```python
from build123d import *

# Parameters (mm, degrees)
SCHIZZO2_R                   = 55.0225
SCHIZZO2_R_2                 = 40.0225
ESTRUSIONE_ESTRUSIONE1_DEPTH = 10
SCHIZZO2_3_R                 = 40.0225
SCHIZZO2_3_R_2               = 25.0225
ESTRUSIONE_ESTRUSIONE2_DEPTH = 15
SCHIZZO2_4_R                 = 25.0225
SCHIZZO2_4_R_2               = 5
ESTRUSIONE_ESTRUSIONE3_DEPTH = 20


with BuildPart() as part:
    # Schizzo2 → Estrusione-Estrusione1 (new body)
    with BuildSketch(Plane(origin=(0, 0, 0), x_dir=(1, 0, 0), z_dir=(0, 1, 0))):
        with Locations(Location((0, 0, 0), (0, 0, 270))):
            Circle(SCHIZZO2_R)
        with Locations(Location((0, 0, 0), (0, 0, 270))):
            Circle(SCHIZZO2_R_2, mode=Mode.SUBTRACT)
    extrude(amount=ESTRUSIONE_ESTRUSIONE1_DEPTH)

    # Schizzo2_3 → Estrusione-Estrusione2 (add)
    with BuildSketch(Plane(origin=(0, 0, 0), x_dir=(1, 0, 0), z_dir=(0, 1, 0))):
        with Locations(Location((0, 0, 0), (0, 0, 270))):
            Circle(SCHIZZO2_3_R)
        with Locations(Location((0, 0, 0), (0, 0, 270))):
            Circle(SCHIZZO2_3_R_2, mode=Mode.SUBTRACT)
    extrude(amount=ESTRUSIONE_ESTRUSIONE2_DEPTH)

    # Schizzo2_4 → Estrusione-Estrusione3 (add)
    with BuildSketch(Plane(origin=(0, 0, 0), x_dir=(1, 0, 0), z_dir=(0, 1, 0))):
        with Locations(Location((0, 0, 0), (0, 0, 270))):
            Circle(SCHIZZO2_4_R)
        with Locations(Location((0, 0, 0), (0, 0, 270))):
            Circle(SCHIZZO2_4_R_2, mode=Mode.SUBTRACT)
    extrude(amount=ESTRUSIONE_ESTRUSIONE3_DEPTH)


solid = part.part
```
CAD build for the part. Positions are in the model's coordinates, mm. A direction names the side the tool comes from. Round coordinates to 2 decimals unless told otherwise and drop trailing zeros. Write each loop counter-clockwise with the first axis right and the second up, starting at its lowest first coordinate (ties: lowest second). Pieces come first, ordered by that corner, then holes.
Item 1: Drop flat-ended pins along their axis: pin 1 Ø6 at (x, y) = (-28, 12.5) entering from +Z; pin 2 Ø1.5 at (y, z) = (4.5, -4.5) entering from -X; pin 3 Ø8 at (y, z) = (10.5, 40) entering from -X. Give the stop position or say it passes through.
Filled in:
pin 1: stops at z = 48.31
pin 2: stops at x = -54.89
pin 3: stops at x = -41.58
Item 2: Band-saw the part on C-C on y = 4.75. Write the cut outline in (x, z) (1 decimal), then the cut area to 3 significant figures.
Filled in:
outline: circle Ø110 at (0, 0); hole circle Ø10 at (0, 0)
area: 9,430 mm2
Item 3: Drill centre lines: L1, parallel to X at y = 7.25, z = 0; L2, parallel to X at y = 10.5, z = 0; L3, parallel to Y at x = 25.5, z = 4. Where is each one in solid material? Low to high.
Filled in:
L1: x = -55.02 to -5, 5 to 55.02
L2: x = -40.02 to -5, 5 to 40.02
L3: y = 0 to 15
Item 4: Band-saw the part on B-B on x = 0. Write the cut outline in (y, z).
Filled in:
outline: (0, -55.02) - (10, -55.02) - (10, -40.02) - (15, -40.02) - (15, -25.02) - (20, -25.02) - (20, -5) - (0, -5) - close; (0, 5) - (20, 5) - (20, 25.02) - (15, 25.02) - (15, 40.02) - (10, 40.02) - (10, 55.02) - (0, 55.02) - close
Item 5: Band-saw the part on D-D on x = 20. Write the cut outline in (y, z).
Filled in:
outline: (0, -51.26) - (10, -51.26) - (10, -34.67) - (15, -34.67) - (15, -15.04) - (20, -15.04) - (20, 15.04) - (15, 15.04) - (15, 34.67) - (10, 34.67) - (10, 51.26) - (0, 51.26) - close
Item 6: Tool access for faces 1 (the cylindrical face through (46.395, 4.93, 29.58)), 2 (the flat face through (-41, 10, 4)): list every direction of +Z, -Z, +X, -X, +Y, -Y with a clear straight run to the whole face (end or side of a thin tool).
Filled in:
face 1: +Y, -Y
face 2: +Y
Item 7: Band-saw the part on A-A on z = 0. Write the cut outline in (x, y).
Filled in:
outline: (-55.02, 0) - (-5, 0) - (-5, 20) - (-25.02, 20) - (-25.02, 15) - (-40.02, 15) - (-40.02, 10) - (-55.02, 10) - close; (5, 0) - (55.02, 0) - (55.02, 10) - (40.02, 10) - (40.02, 15) - (25.02, 15) - (25.02, 20) - (5, 20) - close
